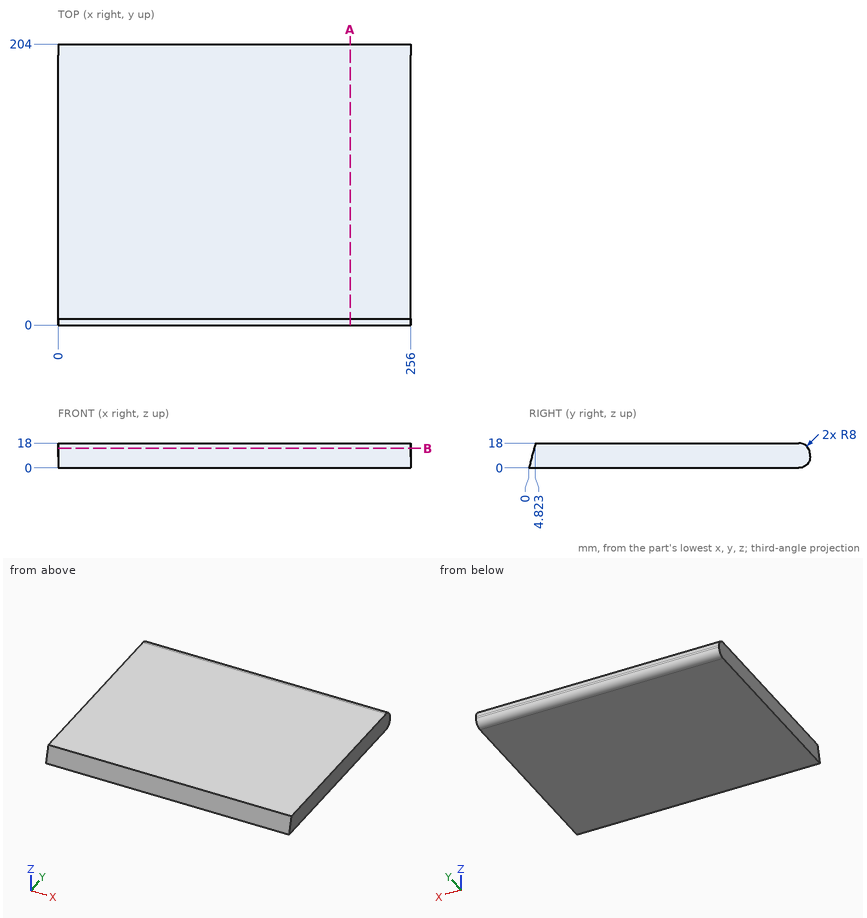
Here's the drawing with two shaded views (mm, measured from the low corner). I have some questions. Coordinates: 2 decimals unless noted, no trailing zeros. Loops run counter-clockwise (first coordinate to the right, second up) from the corner with the lowest first, then second, coordinate; pieces in that order, holes last. Notation, with made-up numbers: (7, 10.5) -> (62, 10.5) arc R11 ccw to (62, 15.5) -> close; hole circle Ø5 at (11.25, -33.5). An arc over 180 degrees is marked (long way). Answer as a JSON object with one key per item and string values.
1) For P1, Ø4, axis at x = 222, z = 9.5, coming from the -Y side; P2, Ø4, axis at x = 50, z = 13, coming from the +Y side; P3, Ø5, axis at x = 139, z = 11, coming from the -Y side, each with a flat end and sliding along its axis, tell me the tip position at first contact or that it passes through.
Results:
{"P1": "stops at y = 2.01", "P2": "stops at y = 203.94", "P3": "stops at y = 2.28"}
2) Imagine slicing it at B-B (z = 14.25). Please give me the cut outline in (x, y).
Results:
{"outline": "(0, 3.82) -> (256, 3.82) -> (256, 202.78) -> (0, 202.78) -> close"}
3) Imagine slicing it at A-A (x = 212). Please give me the cut outline in (y, z).
Results:
{"outline": "(0, 0) -> (196, 0) arc R8 ccw to (204, 8) -> (204, 10) arc R8 ccw to (196, 18) -> (4.82, 18) -> close"}
4) If I drill on line 1 (Y direction, x = 71.5, z = 5.25); line 2 (Y direction, x = 144, z = 11.5), over which ranges is the centre line in solid material (lowest first)?
Results:
{"line 1": "y = 1.41 to 203.51", "line 2": "y = 3.08 to 203.86"}
